```python
from build123d import *

# Parameters (mm, degrees)
F0_R     = 5.5
F0_R_2   = 4.45
F1_DEPTH = 5
F3_DEPTH = 2
F4_DEPTH = 2
F5_SIZE  = 1
F6_SIZE  = 0.5
F7_SIZE  = 0.3
F8_R     = 1


with BuildPart() as f1:
    # F0 (on Top) → F1 (new body)
    with BuildSketch(Plane.XY):
        Circle(F0_R)
        Circle(F0_R_2, mode=Mode.SUBTRACT)
    extrude(amount=F1_DEPTH)

    # F2 (on face) → F3 (join)
    with BuildSketch(Plane.XY.offset(5)):
        with BuildLine():
            Line((-3.2322592718, -4.45), (0, -4.45))
            ThreePointArc((0, -4.45), (-4.45, 0), (0, 4.45))
            Line((0, 4.45), (-3.2322592718, 4.45))
            ThreePointArc((-3.2322592718, 4.45), (-5.5, 0), (-3.2322592718, -4.45))
        make_face()
        with BuildLine():
            Line((0, -4.45), (3.2322592718, -4.45))
            ThreePointArc((3.2322592718, -4.45), (4.9003788626, -2.4972558945), (5.5, 0))
            ThreePointArc((5.5, 0), (4.9003788626, 2.4972558945), (3.2322592718, 4.45))
            Line((3.2322592718, 4.45), (0, 4.45))
            ThreePointArc((0, 4.45), (3.1466251763, 3.1466251763), (4.45, 0))
            ThreePointArc((4.45, 0), (3.1466251763, -3.1466251763), (0, -4.45))
        make_face()
        with BuildLine():
            Line((-6.5, -4.45), (-3.2322592718, -4.45))
            ThreePointArc((-3.2322592718, -4.45), (-5.5, 0), (-3.2322592718, 4.45))
            Line((-3.2322592718, 4.45), (-6.5, 4.45))
            Line((-6.5, 4.45), (-6.5, -4.45))
        make_face()
        with BuildLine():
            Line((3.2322592718, -4.45), (6.5, -4.45))
            Line((6.5, -4.45), (6.5, 4.45))
            Line((6.5, 4.45), (3.2322592718, 4.45))
            ThreePointArc((3.2322592718, 4.45), (4.9003788626, 2.4972558945), (5.5, 0))
            ThreePointArc((5.5, 0), (4.9003788626, -2.4972558945), (3.2322592718, -4.45))
        make_face()
    extrude(amount=-F3_DEPTH)

    # F2 (on face) → F4 (join, symmetric)
    with BuildSketch(Plane.XY.offset(5)):
        with BuildLine():
            Line((6.5, 4.45), (6.5, -4.45))
            Line((6.5, -4.45), (6.5, -6.45))
            Line((6.5, -6.45), (8.5, -6.45))
            Line((8.5, -6.45), (8.5, 6.45))
            Line((8.5, 6.45), (-8.5, 6.45))
            Line((-8.5, 6.45), (-8.5, -6.45))
            Line((-8.5, -6.45), (-6.5, -6.45))
            Line((-6.5, -6.45), (-6.5, -4.45))
            Line((-6.5, -4.45), (-6.5, 4.45))
            Line((-6.5, 4.45), (-3.2322592718, 4.45))
            ThreePointArc((-3.2322592718, 4.45), (0, 5.5), (3.2322592718, 4.45))
            Line((3.2322592718, 4.45), (6.5, 4.45))
        make_face()
        with BuildLine():
            Line((6.5, -6.45), (6.5, -4.45))
            Line((6.5, -4.45), (3.2322592718, -4.45))
            ThreePointArc((3.2322592718, -4.45), (0, -5.5), (-3.2322592718, -4.45))
            Line((-3.2322592718, -4.45), (-6.5, -4.45))
            Line((-6.5, -4.45), (-6.5, -6.45))
            Line((-6.5, -6.45), (6.5, -6.45))
        make_face()
    extrude(amount=F4_DEPTH, both=True)

    # F5
    f5_edges = [f1.edges().sort_by_distance(p)[0] for p in [
        (-4.86613, -4.45, 7),
        (4.86613, -4.45, 7),
    ]]
    chamfer(f5_edges, length=F5_SIZE)

    # F6
    f6_edges = [f1.edges().sort_by_distance(p)[0] for p in [
        (-4.86613, 4.45, 7),
        (-6.5, 0, 7),
        (6.5, 0, 7),
        (4.86613, 4.45, 7),
    ]]
    chamfer(f6_edges, length=F6_SIZE)

    # F7
    f7_edges = [f1.edges().sort_by_distance(p)[0] for p in [
        (-4.45, 0, 0),
    ]]
    chamfer(f7_edges, length=F7_SIZE)

    # F8
    f8_edges = [f1.edges().sort_by_distance(p)[0] for p in [
        (-8.5, -6.45, 5),
        (8.5, -6.45, 5),
        (8.5, 6.45, 5),
        (-8.5, 6.45, 5),
    ]]
    fillet(f8_edges, radius=F8_R)


solid = f1.part
```
Check sheet for the modelled part. Datum: model origin and axes. Units: mm. A direction names the side the tool comes from. Coordinates: 2 decimals unless noted, no trailing zeros. Order: outer loops, then holes, each group sorted by start corner. A loop starts at its lowest first (then second) coordinate and runs counter-clockwise, first axis right, second up. Notation, with made-up numbers: M 60,74 L 68,74 A31 cw 68,105 Z; hole C -5.75,68 d1. An arc over 180 degrees is marked long. One line per question, with ' | ' between items. Start each with the question number.
Item 1: Access from +Z, -Z, +X, -X, +Y, -Y to the whole of each face (thin tool, end or side, straight path). Record for faces 1 (the flat face through (5, 4.45, 6)), 2 (the flat face through (-6, 0, 3)), 3 (the cylindrical face through (-8.215, -6.149, 5.028)).
Item 2: Gauge pin test, flat end, axial feed: P1, Ø1.5, axis at x = 1.5, y = -3.5, coming from the -Z side. Record the tip position at first contact, or that the pin passes through.
Item 3: Material ranges on line 1 (X direction, y = 0, z = 1.85); line 2 (X direction, y = -1.25, z = 5.25); line 3 (Z direction, x = 2.75, y = -4.25), recorded low to high.
Item 4: Sectioned sample at C-C on x = 0. Record the cut outline in (y, z).
Item 5: Sectioned sample at A-A on y = 0. Record the cut outline in (x, z), and give its area (3 significant figures).
Item 6: Sectioned sample at D-D on x = -5. Record the cut outline in (y, z), and give its area (3 significant figures).
Item 7: Sectioned sample at B-B on z = 4.75. Record the cut outline in (x, y).
Answer below:
1) face 1: +Z | face 2: -Z | face 3: +Z, -Z, -X, -Y
2) P1: stops at z = 0.19
3) line 1: x = -5.5 to -4.45, 4.45 to 5.5 | line 2: x = -8.5 to -6.5, 6.5 to 8.5 | line 3: z = 0 to 5
4) outline: M -6.45,3 L -5.5,3 L -5.5,0 L -4.75,0 L -4.45,0.3 L -4.45,5 L -5.5,5 L -5.5,7 L -6.45,7 Z; M 4.45,0.3 L 4.75,0 L 5.5,0 L 5.5,3 L 6.45,3 L 6.45,7 L 5.5,7 L 5.5,5 L 4.45,5 Z
5) outline: M -8.5,3 L -5.5,3 L -5.5,0 L -4.75,0 L -4.45,0.3 L -4.45,5 L -6.5,5 L -6.5,6.5 L -7,7 L -8.5,7 Z; M 4.45,0.3 L 4.75,0 L 5.5,0 L 5.5,3 L 8.5,3 L 8.5,7 L 7,7 L 6.5,6.5 L 6.5,5 L 4.45,5 Z | area: 30.2 mm^2
6) outline: M -6.45,3 L -2.29,3 L -2.29,0 L 2.29,0 L 2.29,3 L 6.45,3 L 6.45,7 L 4.95,7 L 4.45,6.5 L 4.45,5 L -4.45,5 L -4.45,6 L -5.45,7 L -6.45,7 Z | area: 46.9 mm^2
7) outline: M -8.5,-5.45 A1 ccw -7.5,-6.45 L 7.5,-6.45 A1 ccw 8.5,-5.45 L 8.5,5.45 A1 ccw 7.5,6.45 L -7.5,6.45 A1 ccw -8.5,5.45 Z; hole C 0,0 d8.9
